Work out the finished part from the listing and answer in its coordinate system (mm). Face numbers are marked on the shaded views. Round coordinates to 2 decimals unless told otherwise and drop trailing zeros. Write each loop counter-clockwise with the first axis right and the second up, starting at its lowest first coordinate (ties: lowest second). Pieces come first, ordered by that corner, then holes. Notation, with made-up numbers: (76.25, 56) -> (118.25, 56) arc R27 ccw to (118.25, 79) -> close; hole circle Ø8 at (75.5, -6.75). An arc over 180 degrees is marked (long way). One line per item, written item: value.
Autodesk Inventor part; units mm, degrees
ref_plane "YZ Plane" through (0, 0, 0) normal (1, 0, 0) x (0, 1, 0)
ref_plane "XZ Plane" through (0, 0, 0) normal (0, 1, 0) x (-1, 0, 0)
ref_plane "XY Plane" through (0, 0, 0) normal (0, 0, 1) x (1, 0, 0)
sketch "Sketch1" plane through (0, 0, 0) normal (0, 0, 1) x (1, 0, 0)
  line L0 (-30, 40) -> (30, 40)
  line L1 (0, 40) -> (0, 10.3) construction
  circle A0 centre (0, 10.3) radius 20
  line L2 (-23.5, -13.2) -> (23.5, -13.2) construction
  line L3 (23.5, -13.2) -> (23.5, 33.8) construction
  line L4 (23.5, 33.8) -> (-23.5, 33.8) construction
  line L5 (-23.5, 33.8) -> (-23.5, -13.2) construction
  line L6 (23.5, -13.2) -> (-23.5, 33.8) construction
  circle A1 centre (-23.5, 33.8) radius 2.55
  circle A2 centre (23.5, 33.8) radius 2.55
  circle A3 centre (-23.5, -13.2) radius 2.55
  circle A4 centre (23.5, -13.2) radius 2.55
  line L7 (0, -46.275) -> (-30, -46.275)
  line L8 (0, -46.275) -> (30, -46.275)
  line L9 (-30, 40) -> (-30, -46.275)
  line L10 (30, 40) -> (30, -46.275)
  point P0 (0, 0)
  dimension "d2" = 29.7
  dimension "d3" = 40
  dimension "d4" = 47
  dimension "d5" = 47
  dimension "d6" = 5.1
  dimension "d7" = 5.1
  dimension "d8" = 5.1
  dimension "d9" = 5.1
  dimension "d12" = 56.575
  dimension "d13" = 30
  dimension "d14" = 30
extrude "Extrusion1" add sketch "Sketch1" along normal blind 3
sketch "Sketch2" plane through (0, 0, 0) normal (0, 0, -1) x (-1, 0, 0)
  line L0 (30, -46.275) -> (-30, -46.275)
  line L1 (-30, -46.275) -> (-30, 40)
  line L2 (30, -46.275) -> (-30, -46.275)
  line L3 (-30, -46.275) -> (-30, -43.275)
  line L4 (-30, -43.275) -> (30, -43.275)
  line L5 (30, -43.275) -> (30, -46.275)
  point P0 (0, 0)
  dimension "d15" = 3
extrude "Extrusion2" add sketch "Sketch2" along normal blind 30
sketch "Sketch3" plane through (-30, -43.275, 0) normal (0, 1, 0) x (1, 0, 0)
  line L0 (60, -3) -> (0, -3) construction
  line L1 (30, -3) -> (30, 17.57) construction
  line L2 (30, -3) -> (30, 10.43) construction
  line L3 (30, 10.43) -> (30, 17.57) construction
  line L4 (30, 14) -> (65.9748, 14) construction
  line L5 (65.9748, 14) -> (-8.6143, 14) construction
  line L6 (10, 14) -> (50, 14) construction
  line L7 (10, 11.25) -> (50, 11.25)
  line L8 (50, 16.75) -> (10, 16.75)
  arc A0 (10, 16.75) -> (10, 11.25) centre (10, 14) ccw
  arc A1 (50, 11.25) -> (50, 16.75) centre (50, 14) ccw
  point P0 (30, 0)
  dimension "d18" = 20.57
  dimension "d19" = 13.43
  dimension "d20" = 20
  dimension "d21" = 5.5
extrude "Extrusion3" cut sketch "Sketch3" against normal through all
properties part number "Nema23MountPlate" material "Aluminum 6061"
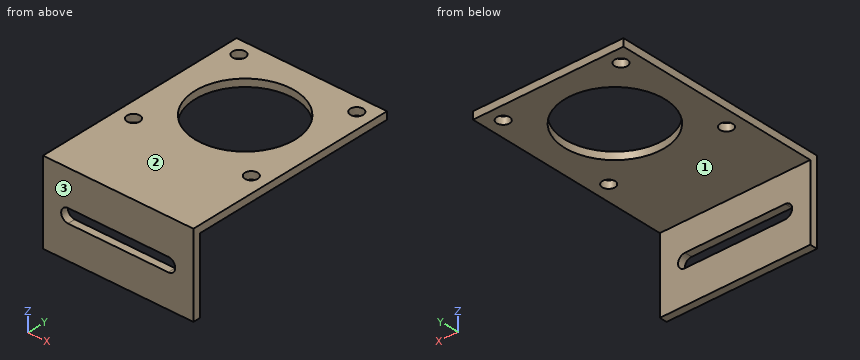
(1) Find section B-B on y = 10.3. Give the vertices of the cut face in (x, z).
Reported:
outline: (-30, 0) -> (-20, 0) -> (-20, 3) -> (-30, 3) -> close; (20, 0) -> (30, 0) -> (30, 3) -> (20, 3) -> close
(2) Consider probe 1 along Y at (x, z) = (-23.5, 1.4) (3 decimals); probe 2 along X at (y, z) = (-13, 2); probe 3 along Y at (x, z) = (0, 1.6) (3 decimals). Determine where each line is inside the solid, lowest interval first.
Reported:
probe 1: y = -46.275 to -15.75, -10.65 to 31.25, 36.35 to 40
probe 2: x = -30 to -26.04, -20.96 to 20.96, 26.04 to 30
probe 3: y = -46.275 to -9.7, 30.3 to 40
(3) Flat-ended cylindrical pins translate along their axes: pin 1 Ø2 at (x, z) = (12, -12) entering from +Y (3 decimals); pin 2 Ø6.5 at (x, y) = (23.5, 33.8) entering from -Z; pin 3 Ø24 at (x, y) = (0, 10.3) entering from -Z. Find the tip coordinate at first contact, or state that the pin passes through.
Reported:
pin 1: stops at y = -43.275
pin 2: stops at z = 0
pin 3: passes through
(4) Find section A-A on y = -13.2. Give the vertices of the cut face in (x, z).
Reported:
outline: (-30, 0) -> (-26.05, 0) -> (-26.05, 3) -> (-30, 3) -> close; (-20.95, 0) -> (20.95, 0) -> (20.95, 3) -> (-20.95, 3) -> close; (26.05, 0) -> (30, 0) -> (30, 3) -> (26.05, 3) -> close
(5) Find section C-C on z = -14. Give the vertices of the cut face in (x, y) (3 decimals), plus the area to 3 significant figures.
Reported:
outline: (-30, -46.275) -> (-22.75, -46.275) -> (-22.75, -43.275) -> (-30, -43.275) -> close; (22.75, -46.275) -> (30, -46.275) -> (30, -43.275) -> (22.75, -43.275) -> close
area: 43.5 mm2
(6) Find section D-D on x = 25. Give the vertices of the cut face in (y, z) (3 decimals).
Reported:
outline: (-46.275, -30) -> (-43.275, -30) -> (-43.275, 0) -> (-15.262, 0) -> (-15.262, 3) -> (-46.275, 3) -> close; (-11.138, 0) -> (31.738, 0) -> (31.738, 3) -> (-11.138, 3) -> close; (35.862, 0) -> (40, 0) -> (40, 3) -> (35.862, 3) -> close
(7) For a pull along Z with two mould halves and no side action, classify the marked faces 1, 2 and 3 as pulls with the +Z half, pulls with the -Z half, needs draft (parallel to the pull), parting line crosses it, or undercut.
Reported:
face 1: pulls with the -Z half
face 2: pulls with the +Z half
face 3: needs draft
